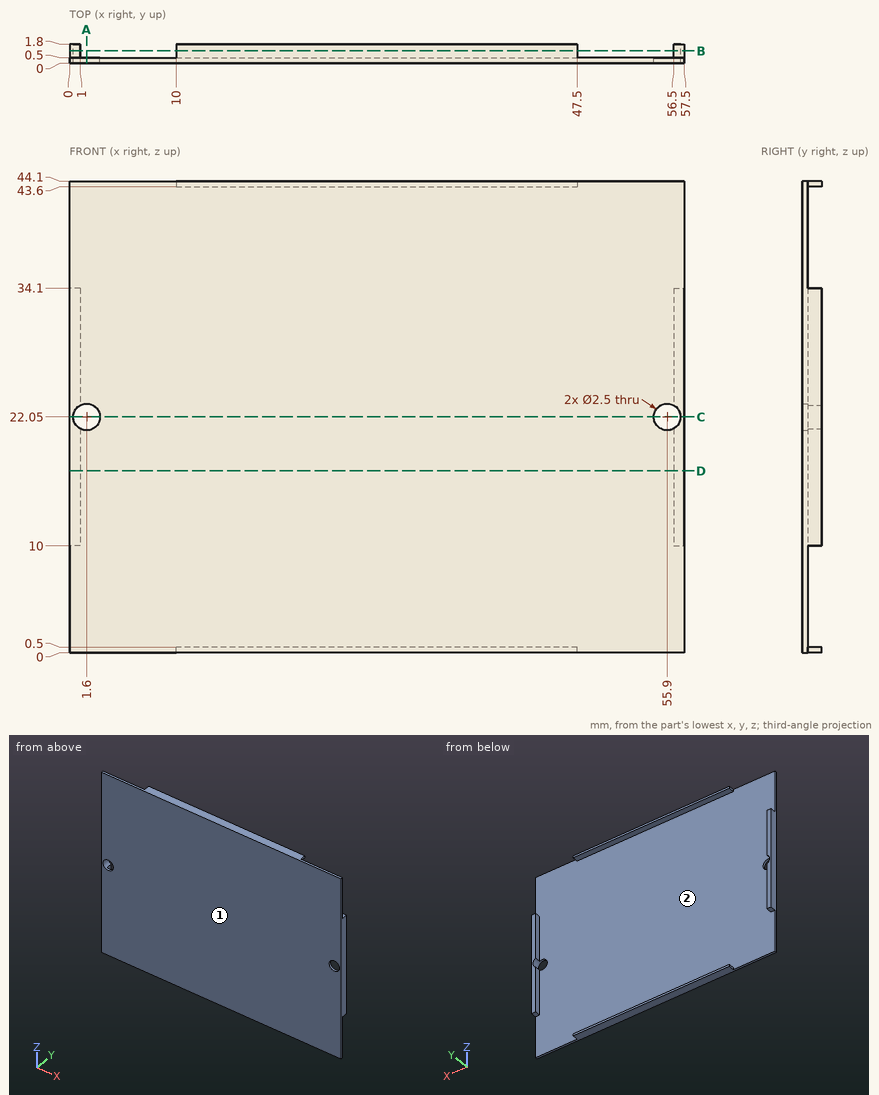
Can you work these out from the drawing? Everything is in mm from the part's minimum corner. Give positions to 0.01 mm unless a question says otherwise; leave off trailing zeros. Order: outer loops, then holes, each group sorted by start corner. A loop starts at its lowest first (then second) coordinate and runs counter-clockwise, first axis right, second up. Notation, with made-up numbers: M -25.5,63.25 L 32.5,63.25 A14 cw 32.5,67.25 Z; hole C 15,-9.75 d5. An arc over 180 degrees is marked long. Use a Markdown table: item, result. Add a question column.
Item 1: Suppose I cut it at C-C (z = 22.05). List the corners of the cut face in (x, y) for me.
Item 2: Suppose I cut it at A-A (x = 1.6). List the corners of the cut face in (y, z) for me, then the cut area to 3 significant figures.
Item 3: Suppose I cut it at D-D (z = 17). List the corners of the cut face in (x, y) for me, then the cut area to 4 significant figures.
Item 4: We'd pull the mould along X, two halves only. Please class the marked faces 1 and 2: +X half, -X half, draft (parallel to the pull), parting line (faces both ways), or undercut.
Item 5: If I drill on L1, parallel to Z at x = 55.9, y = 0.4; L2, parallel to X at y = 0.55, z = 22.05; L3, parallel to Y at x = 42.5, z = 26.5, over which ranges is the centre line in solid material (lowest first)? Write a range as [from, to].
Item 6: Will this pin go through, and if not, where does the flat tip stop? pin 1 (8 mm diameter, centred on x = 19, z = 12.5, fed in from +Y).
Item 7: Suppose I cut it at B-B (y = 1.15). List the corners of the cut face in (x, z) for me.
Answer sheet:
| question | item | result |
|---|---|---|
| 1 | outline | M 0,0 L 0.35,0 L 0.35,1.8 L 0,1.8 Z; M 2.85,0 L 54.65,0 L 54.65,0.5 L 2.85,0.5 Z; M 57.15,0 L 57.5,0 L 57.5,1.8 L 57.15,1.8 Z |
| 2 | outline | M 0,0 L 0.5,0 L 0.5,20.8 L 0,20.8 Z; M 0,23.3 L 0.5,23.3 L 0.5,44.1 L 0,44.1 Z |
| 2 | area | 20.8 mm² |
| 3 | outline | M 0,0 L 57.5,0 L 57.5,1.8 L 56.5,1.8 L 56.5,0.5 L 1,0.5 L 1,1.8 L 0,1.8 Z |
| 3 | area | 31.35 mm² |
| 4 | face 1 | draft |
| 4 | face 2 | undercut |
| 5 | L1 | z = [0, 20.8], [23.3, 44.1] |
| 5 | L2 | x = [0, 0.35], [57.15, 57.5] |
| 5 | L3 | y = [0, 0.5] |
| 6 | pin 1 | stops at y = 0.5 |
| 7 | outline | M 0,10 L 1,10 L 1,20.95 A1.25 cw 1,23.15 L 1,34.1 L 0,34.1 Z; M 10,0 L 47.5,0 L 47.5,0.5 L 10,0.5 Z; M 10,43.6 L 47.5,43.6 L 47.5,44.1 L 10,44.1 Z; M 56.5,10 L 57.5,10 L 57.5,34.1 L 56.5,34.1 L 56.5,23.15 A1.25 cw 56.5,20.95 Z |
